Geometry: final body of the model. Coordinates: model frame, mm. Face numbers are marked on the shaded views. A direction names the side the tool comes from. Give positions to 0.01 mm unless a question says otherwise; leave off trailing zeros. Order: outer loops, then holes, each group sorted by start corner. A loop starts at its lowest first (then second) coordinate and runs counter-clockwise, first axis right, second up. Notation, with made-up numbers: (-4, 21) -> (38, 21) arc R20 cw to (38, 44) -> close; hole circle Ø1 at (70.5, 83). An arc over 180 degrees is marked (long way). Write item = value, one per line.
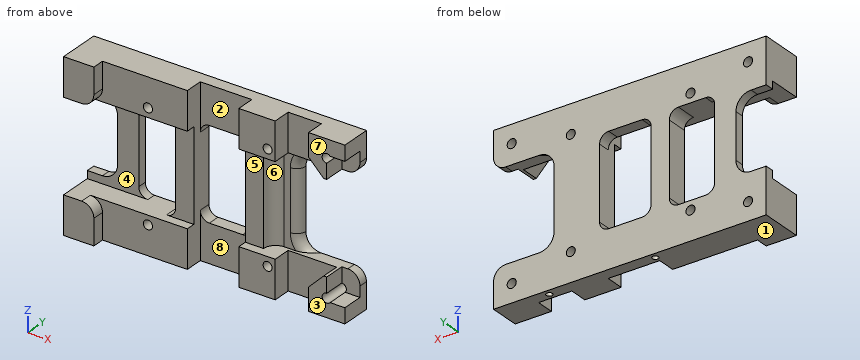
```python
from build123d import *

# Parameters (mm, degrees)
SKETCH_1_W           = 90
SKETCH_1_H           = 55
EXTRUDE_1_DEPTH      = 10
SKETCH_2_R           = 1.5
SKETCH_2_R_2         = 1.48
CUT_EXTRUDE_1_DEPTH  = 30
SKETCH_3_W           = 80
SKETCH_3_H           = 30
SKETCH_3_W_2         = 6
SKETCH_3_H_2         = 45
CUT_EXTRUDE_2_DEPTH  = 7
SKETCH_4_R           = 1.5
CUT_EXTRUDE_3_DEPTH  = 20
SKETCH_8_W           = 10
SKETCH_8_H           = 25
SKETCH_8_W_2         = 20
SKETCH_8_H_2         = 30
CUT_EXTRUDE_6_DEPTH  = 20
SKETCH_10_W          = 11
SKETCH_10_H          = 55
SKETCH_10_W_2        = 17
CUT_EXTRUDE_8_DEPTH  = 6
FILLET_3_R           = 5
SKETCH_11_W          = 6
SKETCH_11_H          = 30
EXTRUDE_3_DEPTH      = 4
CHAMFER_3_SIZE       = 5
FILLET_7_R           = 3
SKETCH_12_W          = 15
SKETCH_12_H          = 30
SKETCH_12_W_2        = 17
CUT_EXTRUDE_9_DEPTH  = 6
FILLET_8_R           = 3
FILLET_9_R           = 4
SKETCH_13_W          = 10
SKETCH_13_H          = 12.5
EXTRUDE_4_DEPTH      = 4
FILLET_10_R          = 4
FILLET_11_R          = 4
SKETCH_14_R          = 1
CUT_EXTRUDE_10_DEPTH = 10


# Some blends are built 0.0001 mm under size
with BuildPart() as part:
    # 草图1 → 凸台-拉伸1 (new body)
    with BuildSketch(Plane(origin=(0, 0, 0), x_dir=(1, 0, 0), z_dir=(0, 1, 0))):
        Rectangle(SKETCH_1_W, SKETCH_1_H)
    extrude(amount=EXTRUDE_1_DEPTH)

    # 草图2 → 切除-拉伸1 (cut)
    with BuildSketch(Plane(origin=(0, 10, 0), x_dir=(1, 0, 0), z_dir=(0, 1, 0))):
        with Locations(Location((-20, 18, 0), (0, 0, 270))):
            Circle(SKETCH_2_R)
        with Locations(Location((-20, -18, 0), (0, 0, 270))):
            Circle(SKETCH_2_R)
        with Locations(Location((19.5, -18.075939793, 0), (0, 0, 270))):
            Circle(SKETCH_2_R_2)
        with Locations(Location((19.5, 18, 0), (0, 0, 270))):
            Circle(SKETCH_2_R_2)
    extrude(amount=-CUT_EXTRUDE_1_DEPTH, mode=Mode.SUBTRACT)

    # 草图3 → 切除-拉伸2 (cut)
    with BuildSketch(Plane.XZ):
        with Locations((-5, 0)):
            Rectangle(SKETCH_3_W, SKETCH_3_H)
        with Locations((42, 0)):
            Rectangle(SKETCH_3_W_2, SKETCH_3_H_2)
    extrude(amount=-CUT_EXTRUDE_2_DEPTH, mode=Mode.SUBTRACT)

    # 草图4 → 切除-拉伸3 (cut)
    with BuildSketch(Plane(origin=(0, 10, 0), x_dir=(1, 0, 0), z_dir=(0, 1, 0))):
        with Locations(Location((39, 21.5, 0), (0, 0, 270))):
            Circle(SKETCH_4_R)
        with Locations(Location((-39, 21.5, 0), (0, 0, 270))):
            Circle(SKETCH_4_R)
        with Locations(Location((-39, -21.5, 0), (0, 0, 270))):
            Circle(SKETCH_4_R)
        with Locations(Location((39, -21.5, 0), (0, 0, 90))):
            Circle(SKETCH_4_R)
    extrude(amount=-CUT_EXTRUDE_3_DEPTH, mode=Mode.SUBTRACT)

    # 草图8 → 切除-拉伸6 (cut)
    with BuildSketch(Plane(origin=(0, 10, 0), x_dir=(1, 0, 0), z_dir=(0, 1, 0))):
        with Locations((-40, 0)):
            Rectangle(SKETCH_8_W, SKETCH_8_H)
        with Locations((35, 0)):
            Rectangle(SKETCH_8_W_2, SKETCH_8_H_2)
    extrude(amount=-CUT_EXTRUDE_6_DEPTH, mode=Mode.SUBTRACT)

    # 草图10 → 切除-拉伸8 (cut)
    with BuildSketch(Plane.XZ):
        with Locations((27.5, 0)):
            Rectangle(SKETCH_10_W, SKETCH_10_H)
        with Locations((1.5, 0)):
            Rectangle(SKETCH_10_W_2, SKETCH_10_H)
    extrude(amount=-CUT_EXTRUDE_8_DEPTH, mode=Mode.SUBTRACT)

    # 圆角3
    fillet_3_edges = [part.edges().sort_by_distance(p)[0] for p in [
        (-35, 8.5, -12.5),
        (-35, 8.5, 12.5),
        (25, 8.5, 15),
        (25, 8.5, -15),
    ]]
    fillet(fillet_3_edges, radius=FILLET_3_R)

    # 草图11 → 凸台-拉伸3 (add)
    with BuildSketch(Plane.XZ.offset(-7)):
        with Locations((-10, 0)):
            Rectangle(SKETCH_11_W, SKETCH_11_H)
        with Locations((13, 0)):
            Rectangle(SKETCH_11_W, SKETCH_11_H)
    extrude(amount=EXTRUDE_3_DEPTH)

    # 倒角3
    chamfer_3_edges = [part.edges().sort_by_distance(p)[0] for p in [
        (33, 3, 15),
        (33, 3, -15),
    ]]
    chamfer(chamfer_3_edges, length=CHAMFER_3_SIZE)

    # 圆角7
    # the kernel refuses this fillet: 3 mm, written as the material it takes off along each edge
    with BuildSketch(Plane(origin=(25, 7, 10), x_dir=(0, 1, 0), z_dir=(0, 0, -1))) as fillet_7_piece_1:
        with BuildLine():
            CenterArc((FILLET_7_R, -FILLET_7_R), FILLET_7_R, 90, 90)
            Line((0, -FILLET_7_R), (0, 0))
            Line((0, 0), (FILLET_7_R, 0))
        make_face()
    extrude(amount=20, mode=Mode.SUBTRACT)
    with BuildSketch(Plane(origin=(30, 7, 10), x_dir=(0.9975374290817743, 0, 0.0701361360564157), z_dir=(0.0701361360564157, 0, -0.9975374290817743))) as fillet_7_piece_2_section:
        with BuildLine():
            CenterArc((5 + FILLET_7_R, -FILLET_7_R), FILLET_7_R, 90, 90)
            Line((5 + FILLET_7_R, 0), (5, 0))
            Line((5, 0), (5, -FILLET_7_R))
        make_face()
    fillet_7_piece_2 = revolve(axis=Axis((30, 7, 10), (0, -1, 0)), revolution_arc=175.978193542, mode=Mode.PRIVATE)
    fillet_7_piece_2 = split(fillet_7_piece_2, bisect_by=Plane(origin=(26.314129742, 7.843114036, 15), z_dir=(0, 0, -1)), keep=Keep.TOP, mode=Mode.PRIVATE)
    add(fillet_7_piece_2, mode=Mode.SUBTRACT)
    with BuildSketch(Plane(origin=(30, 7, -10), x_dir=(0.9975374290817743, 0, -0.0701361360564157), z_dir=(0.0701361360564157, 0, 0.9975374290817743))) as fillet_7_piece_3_section:
        with BuildLine():
            CenterArc((5 + FILLET_7_R, FILLET_7_R), FILLET_7_R, 180, 90)
            Line((5 + FILLET_7_R, 0), (5, 0))
            Line((5, 0), (5, FILLET_7_R))
        make_face()
    fillet_7_piece_3 = revolve(axis=Axis((30, 7, -10), (0, 1, 0)), revolution_arc=175.978193542, mode=Mode.PRIVATE)
    fillet_7_piece_3 = split(fillet_7_piece_3, bisect_by=Plane(origin=(26.31413004, 7.843114018, -15), z_dir=(0, 0, 1)), keep=Keep.TOP, mode=Mode.PRIVATE)
    add(fillet_7_piece_3, mode=Mode.SUBTRACT)

    # 草图12 → 切除-拉伸9 (cut)
    with BuildSketch(Plane.XZ.offset(-7)):
        with Locations((-20.5, 0)):
            Rectangle(SKETCH_12_W, SKETCH_12_H)
        with Locations((1.5, 0)):
            Rectangle(SKETCH_12_W_2, SKETCH_12_H)
    extrude(amount=-CUT_EXTRUDE_9_DEPTH, mode=Mode.SUBTRACT)

    # 圆角8
    fillet_8_edges = [part.edges().sort_by_distance(p)[0] for p in [
        (-7, 8, -15),
        (-7, 8, 15),
        (-13, 6.5, 15),
        (-13, 6.5, -15),
        (10, 8, 15),
        (10, 8, -15),
        (-28, 8.5, -15),
        (-28, 8.5, 15),
    ]]
    fillet(fillet_8_edges, radius=FILLET_8_R)

    # 圆角9
    fillet_9_edges = [part.edges().sort_by_distance(p)[0] for p in [
        (16, 7, 0),
    ]]
    fillet(fillet_9_edges, radius=FILLET_9_R - 0.0001)  # a hair under: the kernel refuses the full size

    # 草图13 → 凸台-拉伸4 (add)
    with BuildSketch(Plane.XZ):
        with Locations((-40, 21.25)):
            Rectangle(SKETCH_13_W, SKETCH_13_H)
        with Locations((-40, -21.25)):
            Rectangle(SKETCH_13_W, SKETCH_13_H)
    extrude(amount=EXTRUDE_4_DEPTH)

    # 圆角10
    fillet_10_edges = [part.edges().sort_by_distance(p)[0] for p in [
        (-35, -2, 15),
        (-35, -2, -15),
    ]]
    fillet(fillet_10_edges, radius=FILLET_10_R)

    # 圆角11
    fillet_11_edges = [part.edges().sort_by_distance(p)[0] for p in [
        (45, 8.5, 15),
        (45, 8.5, -15),
    ]]
    fillet(fillet_11_edges, radius=FILLET_11_R)

    # 草图14 → 切除-拉伸10 (cut)
    with BuildSketch(Plane(origin=(0, 0, -27.5), x_dir=(-1, 0, 0), z_dir=(0, 0, -1))):
        with Locations((-28, 8)):
            Circle(SKETCH_14_R)
        with Locations((7, 8)):
            Circle(SKETCH_14_R)
    extrude(amount=-CUT_EXTRUDE_10_DEPTH, mode=Mode.SUBTRACT)


solid = part.part
```
1) Section query B-B (x = -1). Output: boundary loops of the cut face in (y, z).
Check sheet entries:
outline = (6, -27.5) -> (10, -27.5) -> (10, -15) -> (6, -15) -> close; (6, 15) -> (10, 15) -> (10, 27.5) -> (6, 27.5) -> close
2) First-contact query: P1, Ø2.5, axis at x = 39, z = -21.5, coming from the -Y side; P2, Ø9.5, axis at x = 36, z = 21, coming from the -Y side; P3, Ø3, axis at x = 12.5, z = -0.5, coming from the -Y side; P4, Ø4, axis at x = -30, z = -6.5, coming from the -Y side. Flat tips, straight axial feed; report the tip coordinate or a pass-through.
Check sheet entries:
P1 = through
P2 = 0
P3 = 3
P4 = 7
3) Mould query, pull axis X, two halves, no side actions, for the marked faces 6, 7 and 8. Classes: +X half, -X half, draft (parallel to the pull), parting line (faces both ways), or undercut.
Check sheet entries:
face_6 = +X half
face_7 = draft
face_8 = undercut
4) Reachability of the marked faces 1, 2, 3, 4 and 5 from +Z, -Z, +X, -X, +Y, -Y: full face, straight path, thin tool, end or side. Return the list, or none.
Check sheet entries:
face_1 = -Z, +X, -X, +Y, -Y
face_2 = +Z, -Z, -Y
face_3 = +Z, -Z, +X, -Y
face_4 = -X, -Y
face_5 = +X, -X, -Y
5) Section query C-C (z = -21.5). Output: boundary loops of the cut face in (x, y), plus the area to 3 significant figures.
Check sheet entries:
outline = (-45, -4) -> (-35, -4) -> (-35, 0) -> (-7, 0) -> (-7, 6) -> (10, 6) -> (10, 0) -> (22, 0) -> (22, 6) -> (33, 6) -> (33, 0) -> (37.5, 0) -> (37.5, 10) -> (-37.5, 10) -> (-37.5, 0) -> (-40.5, 0) -> (-40.5, 10) -> (-45, 10) -> close; (40.5, 7) -> (45, 7) -> (45, 10) -> (40.5, 10) -> close; hole circle Ø2 at (-7, 8); hole circle Ø2 at (28, 8)
area = 674 mm²
6) Section query D-D (y = -2.75). Output: boundary loops of the cut face in (x, z).
Check sheet entries:
outline = (-45, -27.5) -> (-35, -27.5) -> (-35, -19) arc R4 ccw to (-39, -15) -> (-45, -15) -> close; (-45, 15) -> (-39, 15) arc R4 ccw to (-35, 19) -> (-35, 27.5) -> (-45, 27.5) -> close
7) Section query A-A (z = 21.5). Output: boundary loops of the cut face in (x, y), plus the area to 4 significant figures.
Check sheet entries:
outline = (-45, -4) -> (-35, -4) -> (-35, 0) -> (-7, 0) -> (-7, 6) -> (10, 6) -> (10, 0) -> (22, 0) -> (22, 6) -> (33, 6) -> (33, 0) -> (37.5, 0) -> (37.5, 10) -> (-37.5, 10) -> (-37.5, 0) -> (-40.5, 0) -> (-40.5, 10) -> (-45, 10) -> close; (40.5, 7) -> (45, 7) -> (45, 10) -> (40.5, 10) -> close
area = 680.5 mm²
8) Line query: line 1 (X direction, y = 6.25, z = -18); line 2 (Z direction, x = -34.5, y = 0.5); line 3 (X direction, y = 9.25, z = 18). Output: solid intervals per line, ascending. Write a range as from..to.
Check sheet entries:
line_1 = -45..-21.5, -18.5..18.02, 20.98..39
line_2 = -27.5..-15, 15..27.5
line_3 = -45..-21.5, -18.5..18.02, 20.98..44.87
